```python
from build123d import *

# Parameters (mm, degrees)
SKETCH1_R           = 2.54
SKETCH1_R_2         = 2.159
BOSS_EXTRUDE1_DEPTH = 3.2004
FILLET1_R           = 6.35
FILLET2_R           = 2.54
SKETCH2_R           = 1.025
CUT_EXTRUDE1_DEPTH  = 3.2004
SKETCH3_W           = 3.81
SKETCH3_H           = 2.54
CUT_EXTRUDE2_DEPTH  = 3.2004


with BuildPart() as part:
    # Sketch1 → Boss-Extrude1 (new body)
    with BuildSketch(Plane.XY):
        with BuildLine():
            Line((15.875, 25.4), (15.875, 9.525))
            Line((15.875, 9.525), (15.875, -17.4625))
            Line((15.875, -17.4625), (-15.875, -17.4625))
            Line((-15.875, -17.4625), (-15.875, 9.525))
            ThreePointArc((-15.875, 9.525), (-11.225320151, 20.750320151), (0, 25.4))
            Line((0, 25.4), (15.875, 25.4))
        make_face()
        Circle(SKETCH1_R, mode=Mode.SUBTRACT)
        with Locations((-9.525, -11.1125)):
            Circle(SKETCH1_R_2, mode=Mode.SUBTRACT)
        with Locations((9.525, -11.1125)):
            Circle(SKETCH1_R_2, mode=Mode.SUBTRACT)
    extrude(amount=BOSS_EXTRUDE1_DEPTH)

    # Fillet1
    fillet1_edges = [part.edges().sort_by_distance(p)[0] for p in [
        (15.875, 25.4, 1.6002),
    ]]
    fillet(fillet1_edges, radius=FILLET1_R)

    # Fillet2
    fillet2_edges = [part.edges().sort_by_distance(p)[0] for p in [
        (15.875, -17.4625, 1.6002),
        (-15.875, -17.4625, 1.6002),
    ]]
    fillet(fillet2_edges, radius=FILLET2_R)

    # Sketch2 → Cut-Extrude1 (cut)
    with BuildSketch(Plane.XY.offset(3.2004)):
        with Locations((-3.7211, 6.44513426)):
            Circle(SKETCH2_R)
        with Locations((3.7211, -6.44513426)):
            Circle(SKETCH2_R)
    extrude(amount=-CUT_EXTRUDE1_DEPTH, mode=Mode.SUBTRACT)

    # Sketch3 → Cut-Extrude2 (cut)
    with BuildSketch(Plane.XY.offset(3.2004)):
        with Locations((4.7625, 21.292785454)):
            Rectangle(SKETCH3_W, SKETCH3_H)
        with Locations((4.7625, 16.212785454)):
            Rectangle(SKETCH3_W, SKETCH3_H)
    extrude(amount=-CUT_EXTRUDE2_DEPTH, mode=Mode.SUBTRACT)


solid = part.part
```
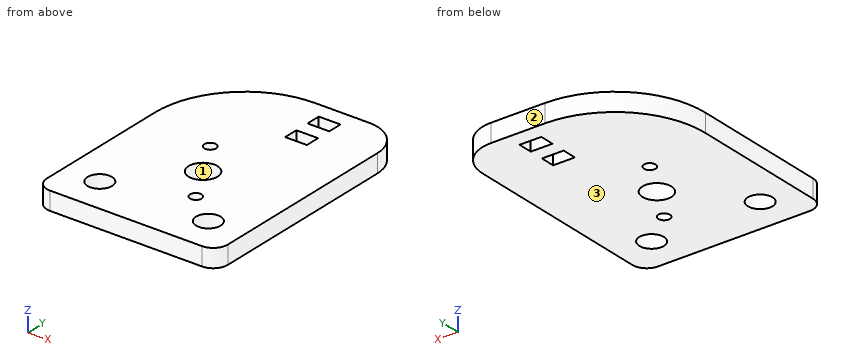
For this review, take the finished solid that the model builds, in its own axes (mm). Face numbers are marked on the shaded views. Coordinates: 2 decimals unless noted, no trailing zeros. Write each loop counter-clockwise with the first axis right and the second up, starting at its lowest first coordinate (ties: lowest second). Pieces come first, ordered by that corner, then holes. Notation, with made-up numbers: (56, -39.5) - (78, -39.5) arc R21 cw to (78, -26.5) - close; hole circle Ø3 at (8, -19). An arc over 180 degrees is marked (long way). Answer in a Markdown table with one row per item. Add a question column.
Q1. For probe 1 along X at (y, z) = (-13, 2.3) (3 decimals); probe 2 along X at (y, z) = (-9.5, 2.55) (3 decimals); probe 3 along Y at (x, z) = (-1.5, 1.5), list the stretches that pass through material, from the lowest coordinate up.
Q2. For P1, Ø3, axis at x = 0, y = 0, coming from the -Z side; P2, Ø1.3, axis at y = 16.5, z = 1, coming from the -X side, all flat-tipped, find the tip position at first contact; note any pin that passes through.
Q3. We need section A-A, the plane y = 0. State the section outline as (x, z) points (3 decimals), and give its area (3 significant figures).
Q4. We need section C-C, the plane x = 3.5. State the section outline as (y, z) points.
Q5. Draft analysis for pull direction Y (two halves, no side actions). For the marked faces 1, 2 and 3, state which applies: +Y half, -Y half, draft (parallel to the pull), parting line (faces both ways), or undercut.
Q6. We need section B-B, the plane z = 1.1. Count the separate pieces of the cut face and the enclosed holes in it, and give its area (3 significant figures).
Answer list:
| question | item | result |
|---|---|---|
| 1 | probe 1 | x = -15.875 to -10.573, -8.477 to 8.477, 10.573 to 15.875 |
| 1 | probe 2 | x = -15.875 to -10.961, -8.089 to 8.089, 10.961 to 15.875 |
| 1 | probe 3 | y = -17.46 to -2.05, 2.05 to 25.33 |
| 2 | P1 | passes through |
| 2 | P2 | stops at x = -14.56 |
| 3 | outline | (-15.875, 0) - (-2.54, 0) - (-2.54, 3.2) - (-15.875, 3.2) - close; (2.54, 0) - (15.875, 0) - (15.875, 3.2) - (2.54, 3.2) - close |
| 3 | area | 85.4 mm2 |
| 4 | outline | (-17.46, 0) - (-7.45, 0) - (-7.45, 3.2) - (-17.46, 3.2) - close; (-5.44, 0) - (14.94, 0) - (14.94, 3.2) - (-5.44, 3.2) - close; (17.48, 0) - (20.02, 0) - (20.02, 3.2) - (17.48, 3.2) - close; (22.56, 0) - (25.4, 0) - (25.4, 3.2) - (22.56, 3.2) - close |
| 5 | face 1 | undercut |
| 5 | face 2 | +Y half |
| 5 | face 3 | draft |
| 6 | separate pieces | 1 |
| 6 | enclosed holes | 7 |
| 6 | area | 1,220 mm2 |
